```python
from build123d import *

# Parameters (mm, degrees)
SKETCH1_W        = 134.3
SKETCH1_H        = 16
STRIP_BASE_DEPTH = 9.5
SKETCH2_R        = 2.5
SCREW_BODY_DEPTH = 2.5
SCREW_START      = -1.3
SCREW_SLOT_DEPTH = 3.8
SKETCH4_W        = 4.3
SKETCH4_H        = 4.3
WIRE_HOLE_DEPTH  = 71.065130414
LPATTERN1_COUNT  = 17
LPATTERN1_PITCH  = 7.5


with BuildPart() as part:
    # Sketch1 → strip base (new, symmetric)
    with BuildSketch(Plane.XY):
        Rectangle(SKETCH1_W, SKETCH1_H)
    extrude(amount=STRIP_BASE_DEPTH, both=True)

    # Sketch2 → screw body (add)
    with BuildSketch(Plane.XY.offset(9.5)):
        with Locations((-60.65, 0)):
            Circle(SKETCH2_R)
    screw_body = extrude(amount=SCREW_BODY_DEPTH)

    # Sketch3 → screw slot (cut)
    with BuildSketch(Plane.XY.offset(12).offset(SCREW_START)):
        Polygon((-58.150833414, 0.653197042), (-63.150829324, 0.646801894), (-63.149166586, -0.653197042), (-58.149170676, -0.646801894), align=None)
    screw_slot = extrude(amount=SCREW_SLOT_DEPTH, mode=Mode.SUBTRACT)

    # Sketch4 → wire hole (cut, through all)
    with BuildSketch(Plane.XZ.offset(8)):
        with Locations((-60.65, 0)):
            Rectangle(SKETCH4_W, SKETCH4_H)
    wire_hole = extrude(amount=-WIRE_HOLE_DEPTH, mode=Mode.SUBTRACT)

    # LPattern1: screw body, screw slot, wire hole ×17
    with Locations(*[(i * LPATTERN1_PITCH, 0, 0) for i in range(1, LPATTERN1_COUNT)]):
        add(screw_body)
        add(screw_slot, mode=Mode.SUBTRACT)
        add(wire_hole, mode=Mode.SUBTRACT)


solid = part.part
```
The model under review builds one solid part; all positions refer to its coordinate system, in mm. A direction names the side the tool comes from. Round coordinates to 2 decimals unless told otherwise and drop trailing zeros. Loops run counter-clockwise (first coordinate to the right, second up) from the corner with the lowest first, then second, coordinate; pieces in that order, holes last. Notation, with made-up numbers: (45.5, 58) -> (58.5, 58) arc R18 cw to (58.5, 84) -> close; hole circle Ø6 at (68, 87.5). An arc over 180 degrees is marked (long way). Answer in a Markdown table with one row per item.
1) Tool access review of faces 3 (the cylindrical face through (16.66, -0.96, 10.73)), 4 (the flat face through (-10.3, 0, 0)): name each direction out of +Z, -Z, +X, -X, +Y, -Y from which nothing blocks a thin tool from reaching the whole face with its end or side.
Taken from the geometry:
| item | result |
|---|---|
| face 3 | +Z |
| face 4 | +Y, -Y |
2) For pin 1 Ø3.5 at (x, y) = (44, 0) entering from +Z; pin 2 Ø1 at (x, y) = (-8, 0) entering from +Z, all flat-tipped, find the tip position at first contact; note any pin that passes through.
Taken from the geometry:
| item | result |
|---|---|
| pin 1 | stops at z = 12 |
| pin 2 | stops at z = 10.7 |
3) Consider section C-C, the plane y = 6. Count the separate pieces of the cut face and the enclosed holes in it, plus the area to 3 significant figures.
Taken from the geometry:
| item | result |
|---|---|
| separate pieces | 1 |
| enclosed holes | 17 |
| area | 2,240 mm² |
4) Consider section A-A, the plane x = 44.35. Write out the cut boundary in (y, z).
Taken from the geometry:
| item | result |
|---|---|
| outline | (-8, -9.5) -> (8, -9.5) -> (8, -2.15) -> (-8, -2.15) -> close; (-8, 2.15) -> (8, 2.15) -> (8, 9.5) -> (2.5, 9.5) -> (2.5, 12) -> (0.65, 12) -> (0.65, 10.7) -> (-0.65, 10.7) -> (-0.65, 12) -> (-2.5, 12) -> (-2.5, 9.5) -> (-8, 9.5) -> close |
5) Wall thickness on line 1 along Z through (x, y) = (-1, 5.5); line 2 along Z through (x, y) = (-10, 0); line 3 along Y through (x, z) = (-46, 10.75): over which ranges is each line inside the solid? List them lowest first.
Taken from the geometry:
| item | result |
|---|---|
| line 1 | z = -9.5 to -2.15, 2.15 to 9.5 |
| line 2 | z = -9.5 to -2.15, 2.15 to 10.7 |
| line 3 | y = -2.48 to -0.65, 0.65 to 2.48 |
6) Consider section D-D, the plane x = -34.5. Write out the cut boundary in (y, z).
Taken from the geometry:
| item | result |
|---|---|
| outline | (-8, -9.5) -> (8, -9.5) -> (8, 9.5) -> (-8, 9.5) -> close |
7) Draft analysis for pull direction X (two halves, no side actions). For faces 1 (the flat face through (54, 0, 0)), 2 (the flat face through (67.15, 0, 0)), state which applies: pulls with the +X half, pulls with the -X half, needs draft (parallel to the pull), parting line crosses it, or undercut.
Taken from the geometry:
| item | result |
|---|---|
| face 1 | undercut |
| face 2 | pulls with the +X half |
